```python
from build123d import *

# Parameters (mm, degrees)
BOSS_EXTRUDE1_DEPTH = 4
BOSS_EXTRUDE2_DEPTH = 2.25
SKETCH3_R           = 7.95
CUT_EXTRUDE1_DEPTH  = 9.25
SKETCH4_R           = 2
CUT_EXTRUDE2_DEPTH  = 9.25
CUT_EXTRUDE3_DEPTH  = 3
FILLET1_R           = 2.36
CHAMFER1_SIZE       = 3.5
CHAMFER1_SIZE2      = 2.020725942
BOSS_EXTRUDE3_DEPTH = 4
FILLET2_R           = 2
SKETCH7_W           = 56.562445917
SKETCH7_H           = 51.963873078
CUT_EXTRUDE4_DEPTH  = 0.1
FILLET3_R           = 2.38


with BuildPart() as part:
    # Sketch1 → Boss-Extrude1 (new body)
    with BuildSketch(Plane(origin=(0, 0, 0), x_dir=(1, 0, 0), z_dir=(0, 1, 0))):
        with BuildLine():
            Line((-13.29118379, 20.889836125), (-0.68999579, 20.889836125))
            Line((-0.68999579, 20.889836125), (-0.68999579, 24.09210312))
            Line((-0.68999579, 24.09210312), (-0.68999579, 26.09210312))
            Line((-0.68999579, 26.09210312), (12.01000421, 26.09210312))
            Line((12.01000421, 26.09210312), (12.01000421, 24.09210312))
            Line((12.01000421, 24.09210312), (12.01000421, -26.90789688))
            Line((12.01000421, -26.90789688), (12.01000421, -28.90789688))
            Line((12.01000421, -28.90789688), (-0.68999579, -28.90789688))
            Line((-0.68999579, -28.90789688), (-0.68999579, -26.90789688))
            Line((-0.68999579, -26.90789688), (-0.68999579, -23.705629885))
            Line((-0.68999579, -23.705629885), (-13.29118379, -23.705629885))
            ThreePointArc((-13.29118379, -23.705629885), (-35.588916795, -1.40789688), (-13.29118379, 20.889836125))
        make_face()
    extrude(amount=BOSS_EXTRUDE1_DEPTH)

    # Sketch2 → Boss-Extrude2 (add)
    with BuildSketch(Plane(origin=(0, 4, 0), x_dir=(1, 0, 0), z_dir=(0, 1, 0))):
        with BuildLine():
            Line((-0.68999579, 20.889836125), (-0.68999579, 16.987726462))
            ThreePointArc((-0.68999579, 16.987726462), (9.006549215, -1.40789688), (-0.68999579, -19.803520222))
            Line((-0.68999579, -19.803520222), (-0.68999579, -23.705629885))
            Line((-0.68999579, -23.705629885), (-13.29118379, -23.705629885))
            ThreePointArc((-13.29118379, -23.705629885), (-35.588916795, -1.40789688), (-13.29118379, 20.889836125))
            Line((-13.29118379, 20.889836125), (-0.68999579, 20.889836125))
        make_face()
    extrude(amount=BOSS_EXTRUDE2_DEPTH)

    # Sketch3 → Cut-Extrude1 (cut)
    with BuildSketch(Plane.XZ):
        with Locations(Location((-13.29118379, 1.40789688, 0), (0, 0, 270))):
            Circle(SKETCH3_R)
    extrude(amount=-CUT_EXTRUDE1_DEPTH, mode=Mode.SUBTRACT)

    # Sketch4 → Cut-Extrude2 (cut)
    with BuildSketch(Plane.XZ):
        with Locations(Location((3.31000421, -21.59210312, 0), (0, 0, 270))):
            Circle(SKETCH4_R)
        with Locations(Location((3.31000421, 24.40789688, 0), (0, 0, 270))):
            Circle(SKETCH4_R)
    extrude(amount=-CUT_EXTRUDE2_DEPTH, mode=Mode.SUBTRACT)

    # Sketch5 → Cut-Extrude3 (cut)
    with BuildSketch(Plane.XZ):
        with BuildLine():
            ThreePointArc((-20.917233099, -7.792422241), (-25.24118379, 1.40789688), (-20.917233099, 10.608216001))
            Line((-20.917233099, 10.608216001), (-24.193916765, 16.291878661))
            ThreePointArc((-24.193916765, 16.291878661), (-31.74118379, 1.40789688), (-24.193916765, -13.476084902))
            Line((-24.193916765, -13.476084902), (-20.917233099, -7.792422241))
        make_face()
        with BuildLine():
            Line((-20.729723635, 18.291931497), (-17.445869217, 12.612408873))
            ThreePointArc((-17.445869217, 12.612408873), (-7.31618379, 11.756900455), (-1.510449053, 3.412089752))
            Line((-1.510449053, 3.412089752), (5.05008903, 3.407949716))
            ThreePointArc((5.05008903, 3.407949716), (-4.06618379, 17.38606558), (-20.729723635, 18.291931497))
        make_face()
        with BuildLine():
            ThreePointArc((-1.510449053, -0.596295992), (-7.31618379, -8.941106696), (-17.445869217, -9.796615113))
            Line((-17.445869217, -9.796615113), (-20.729723635, -15.476137738))
            ThreePointArc((-20.729723635, -15.476137738), (-4.06618379, -14.57027182), (5.05008903, -0.592155956))
            Line((5.05008903, -0.592155956), (-1.510449053, -0.596295992))
        make_face()
    extrude(amount=-CUT_EXTRUDE3_DEPTH, mode=Mode.SUBTRACT)

    # Fillet1
    fillet1_edges = [part.edges().sort_by_distance(p)[0] for p in [
        (-20.917233099, 1.5, 10.608216001),
        (-20.917233099, 1.5, -7.792422241),
        (-24.193916765, 1.5, -13.476084902),
        (-24.193916765, 1.5, 16.291878661),
        (5.05008903, 1.5, 3.407949716),
        (-1.510449053, 1.5, 3.412089752),
        (-17.445869217, 1.5, 12.612408873),
        (-20.729723635, 1.5, 18.291931497),
        (-17.445869217, 1.5, -9.796615113),
        (-1.510449053, 1.5, -0.596295992),
        (5.05008903, 1.5, -0.592155956),
        (-20.729723635, 1.5, -15.476137738),
    ]]
    fillet(fillet1_edges, radius=FILLET1_R)

    # Chamfer1
    chamfer1_edges = [part.edges().sort_by_distance(p)[0] for p in [
        (12.01000421, 0, 1.40789688),
    ]]
    chamfer1_side = [part.faces().sort_by_distance(p)[0] for p in [
        (-3.702499267, 0, 18.015985651),
    ]]
    chamfer(chamfer1_edges, length=CHAMFER1_SIZE, length2=CHAMFER1_SIZE2, reference=chamfer1_side[0])

    # Sketch6 → Boss-Extrude3 (add)
    with BuildSketch(Plane.XZ):
        with BuildLine():
            Line((-0.68999579, -22.889836125), (-13.29118379, -22.889836125))
            ThreePointArc((-13.29118379, -22.889836125), (-37.588916795, 1.40789688), (-13.29118379, 25.705629885))
            Line((-13.29118379, 25.705629885), (-0.68999579, 25.705629885))
            Line((-0.68999579, 25.705629885), (-0.68999579, 23.705629885))
            Line((-0.68999579, 23.705629885), (-13.29118379, 23.705629885))
            ThreePointArc((-13.29118379, 23.705629885), (-35.588916795, 1.40789688), (-13.29118379, -20.889836125))
            Line((-13.29118379, -20.889836125), (-0.68999579, -20.889836125))
            Line((-0.68999579, -20.889836125), (-0.68999579, -22.889836125))
        make_face()
    extrude(amount=-BOSS_EXTRUDE3_DEPTH)

    # Fillet2
    fillet2_edges = [part.edges().sort_by_distance(p)[0] for p in [
        (-6.99058979, 0, 25.705629885),
        (-37.588916795, 0, 1.40789688),
        (-6.99058979, 0, -22.889836125),
    ]]
    fillet(fillet2_edges, radius=FILLET2_R)

    # Sketch7 → Cut-Extrude4 (cut)
    with BuildSketch(Plane(origin=(0, 6.25, 0), x_dir=(1, 0, 0), z_dir=(0, 1, 0))):
        with Locations((-12.789456293, -2.500057929)):
            Rectangle(SKETCH7_W, SKETCH7_H)
    extrude(amount=-CUT_EXTRUDE4_DEPTH, mode=Mode.SUBTRACT)

    # Fillet3
    fillet3_edges = [part.edges().sort_by_distance(p)[0] for p in [
        (-0.68999579, 5.075, -16.987726462),
        (-0.68999579, 5.075, 19.803520222),
    ]]
    fillet(fillet3_edges, radius=FILLET3_R)


solid = part.part
```
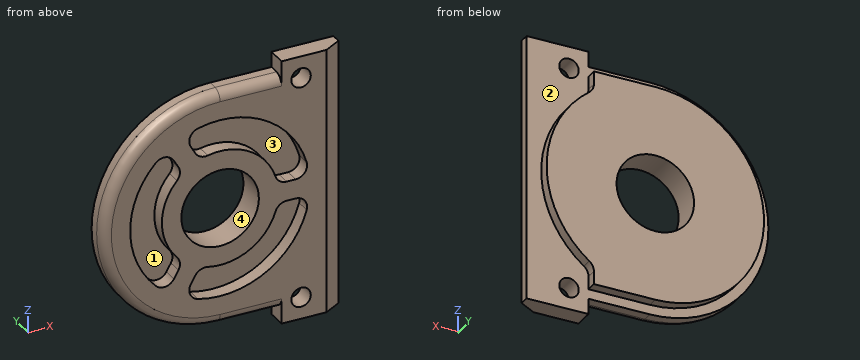
Verification items for the finished model (mm, model axes). Face numbers are marked on the shaded views. A direction names the side the tool comes from. Coordinates: 2 decimals unless noted, no trailing zeros. Write each loop counter-clockwise with the first axis right and the second up, starting at its lowest first coordinate (ties: lowest second). Pieces come first, ordered by that corner, then holes. Notation, with made-up numbers: M -10,-13.5 L 25,-13.5 A18 ccw 25,19.5 Z; hole C -11.5,-1 d5. An arc over 180 degrees is marked long. One line per item, written item: value.
Item 1: Mould release check, pull along Z, two halves, no side actions. Record for the marked faces 1 and 2: pulls with the +Z half, pulls with the -Z half, needs draft (parallel to the pull), parting line crosses it, or undercut.
Check sheet entries:
face 1: undercut
face 2: needs draft
Item 2: Access from +Z, -Z, +X, -X, +Y, -Y to the whole of each face (thin tool, end or side, straight path). Record for the marked faces 3 and 4.
Check sheet entries:
face 3: -Y
face 4: +Y, -Y
Item 3: Section check B-B, the plane x = -12. Record the boundary of the cut face in (y, z), plus the area to 3 significant figures.
Check sheet entries:
outline: M 0,-20.89 A2 ccw 2,-22.89 L 4,-22.89 L 4,-20.89 L 6.15,-20.89 L 6.15,-6.44 L 0,-6.44 L 0,-10.47 L 3,-10.47 L 3,-17 L 0,-17 Z; M 0,9.25 L 6.15,9.25 L 6.15,23.71 L 4,23.71 L 4,25.71 L 2,25.71 A2 ccw 0,23.71 L 0,19.81 L 3,19.81 L 3,13.29 L 0,13.29 Z
area: 153 mm^2
Item 4: Section check C-C, the plane y = 0.75. State how many separate pieces and enclosed holes the cut face has, plus the area to 3 significant figures.
Check sheet entries:
separate pieces: 1
enclosed holes: 6
area: 1,320 mm^2
Item 5: Scan lines: line 1 along X through (y, z) = (1, -5); line 2 along X through (y, z) = (2, 14); line 3 along Z through (x, y) = (-18, 1). Record each from-to range of solid material in increasing order.
Check sheet entries:
line 1: x = -36.45 to -30.59, -23.38 to -18, -8.59 to -3.2, 4.01 to 10.24
line 2: x = -34.07 to -26.78, -22.88 to -18.23, 0.19 to 11.97
line 3: z = -22.16 to -16.43, -10.91 to -5, 7.81 to 13.73, 19.24 to 24.97
Item 6: Section check A-A, the plane y = 4.75. Record the boundary of the cut face in (x, z), plus the area to 3 significant figures.
Check sheet entries:
outline: M -13.29,-20.89 L -0.69,-20.89 L -0.69,-18.2 A2.38 cw 0.25,-16.31 A22.3 ccw 0.25,19.13 A2.38 cw -0.69,21.02 L -0.69,23.71 L -13.29,23.71 A22.3 ccw Z; hole C -13.29,1.41 d15.9
area: 1,400 mm^2
Item 7: Gauge pin test, flat ends, axial feed: pin 1 Ø3 at (y, z) = (2, -14) entering from -X; pin 2 Ø6.5 at (x, z) = (3.31, -21.59) entering from +Y; pin 3 Ø0.6 at (y, z) = (5, -19) entering from +X; pin 4 Ø1.7 at (y, z) = (4.5, 22.5) entering from +X. Record the tip position at first contact, or that the pin passes through.
Check sheet entries:
pin 1: stops at x = -33.21
pin 2: stops at y = 4
pin 3: stops at x = -0.69
pin 4: stops at x = 12.01
